Can you work these out from the drawing? Everything is in mm from the part's minimum corner. Coordinates: 2 decimals unless noted, no trailing zeros. Order: outer loops, then holes, each group sorted by start corner. A loop starts at its lowest first (then second) coordinate and runs counter-clockwise, first axis right, second up. Notation, with made-up numbers: (51.25, 12.25) - (102.25, 12.25) arc R17 ccw to (102.25, 16.25) - close; hole circle Ø8 at (8, 79). An arc over 180 degrees is marked (long way). One line per item, written item: value.
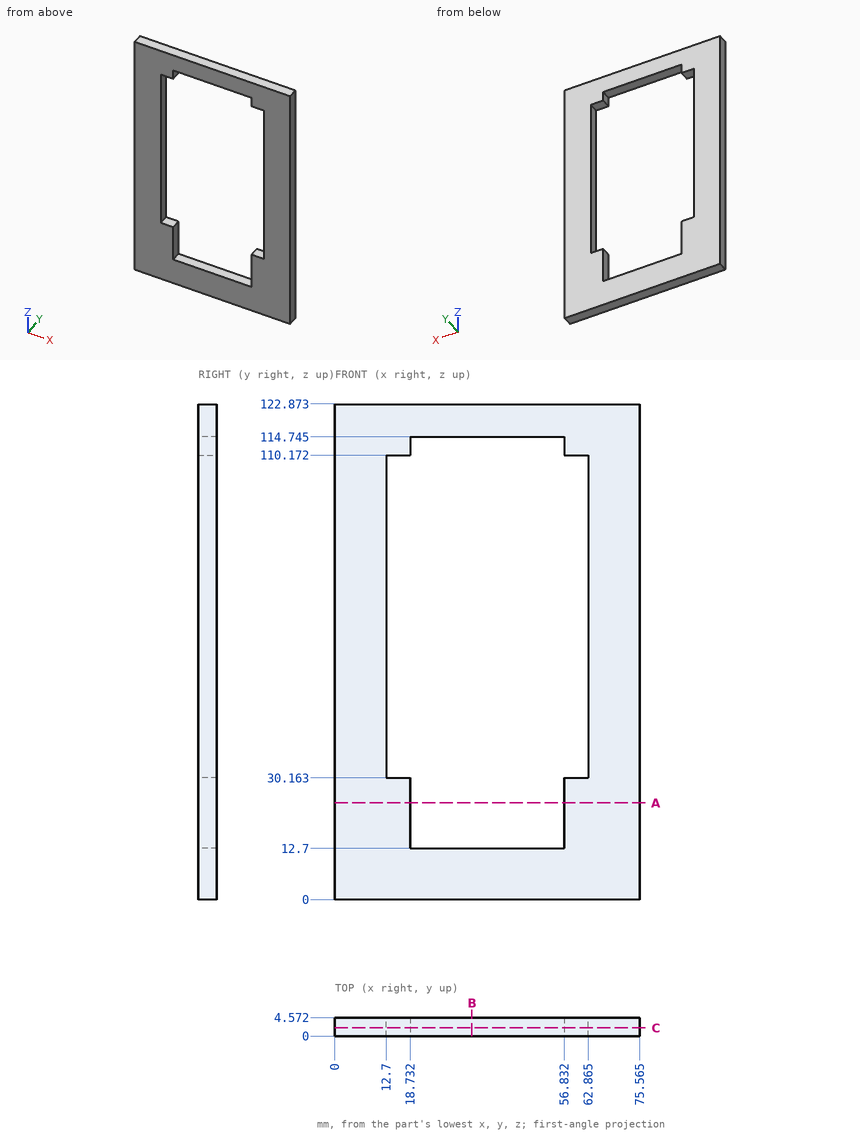
Item 1: I want a section at C-C on y = 2. Please give me the cut outline in (x, z) (1 decimal), then the cut area to 3 significant figures.
Conclusion:
outline: (0, 0) - (75.6, 0) - (75.6, 122.9) - (0, 122.9) - close; hole (12.7, 30.2) - (18.7, 30.2) - (18.7, 12.7) - (56.8, 12.7) - (56.8, 30.2) - (62.9, 30.2) - (62.9, 110.2) - (56.8, 110.2) - (56.8, 114.7) - (18.7, 114.7) - (18.7, 110.2) - (12.7, 110.2) - close
area: 4,430 mm²
Item 2: If I drill on probe 1 along X at (y, z) = (3.6, 53) (1 decimal); probe 2 along Z at (x, y) = (45.5, 1.5) (1 decimal); probe 3 along X at (y, z) = (1.3, 17) (1 decimal), over which ranges is the centre line in solid material (lowest first)?
Conclusion:
probe 1: 0 to 12.7, 62.9 to 75.6
probe 2: 0 to 12.7, 114.7 to 122.9
probe 3: 0 to 18.7, 56.8 to 75.6
Item 3: I want a section at A-A on z = 24. Please give me the cut outline in (x, y) (1 decimal).
Conclusion:
outline: (0, 0) - (18.7, 0) - (18.7, 4.6) - (0, 4.6) - close; (56.8, 0) - (75.6, 0) - (75.6, 4.6) - (56.8, 4.6) - close
Item 4: I want a section at B-B on x = 34. Please give me the cut outline in (y, z) (1 decimal).
Conclusion:
outline: (0, 0) - (4.6, 0) - (4.6, 12.7) - (0, 12.7) - close; (0, 114.7) - (4.6, 114.7) - (4.6, 122.9) - (0, 122.9) - close
